Part print with two shaded views. Sizes in mm from the minimum x, y, z corner. Give positions to 0.01 mm unless a question says otherwise; leave off trailing zeros. Loops run counter-clockwise (first coordinate to the right, second up) from the corner with the lowest first, then second, coordinate; pieces in that order, holes last. Notation, with made-up numbers: (78.5, 27.25) -> (103.5, 27.25) arc R28 cw to (103.5, 64.25) -> close; hole circle Ø1 at (85.5, 68). An arc over 180 degrees is marked (long way). One line per question, with ' | ' between items. Start each with the question number.
(1) Slice it at D-D, the plane x = 38. Write the cut outline in (y, z), then the cut area to 3 significant figures.
(2) Drill centre lines: L1, parallel to Z at x = 22.5, y = 1.2; L2, parallel to Z at x = 7, y = 1.4; L3, parallel to Z at x = 42, y = 2.1 (1 decimal). Where is each one in solid material? Low to high. Write a range as from..to.
(3) Slice it at B-B, the plane y = 2.45. Write the cut outline in (x, z).
(4) Slice it at C-C, the plane z = 7. Write the cut outline in (x, y) (1 decimal).
(5) Flat gauge pins, fed straight in: pin 1 Ø6.5 at (x, z) = (22.5, 8.55) entering from +Y; pin 2 Ø1 at (x, y) = (10, 2.5) entering from +Z. Where does each tip first touch, or does it go through?
(6) Slice it at A-A, the plane x = 22.5. Write the cut outline in (y, z).
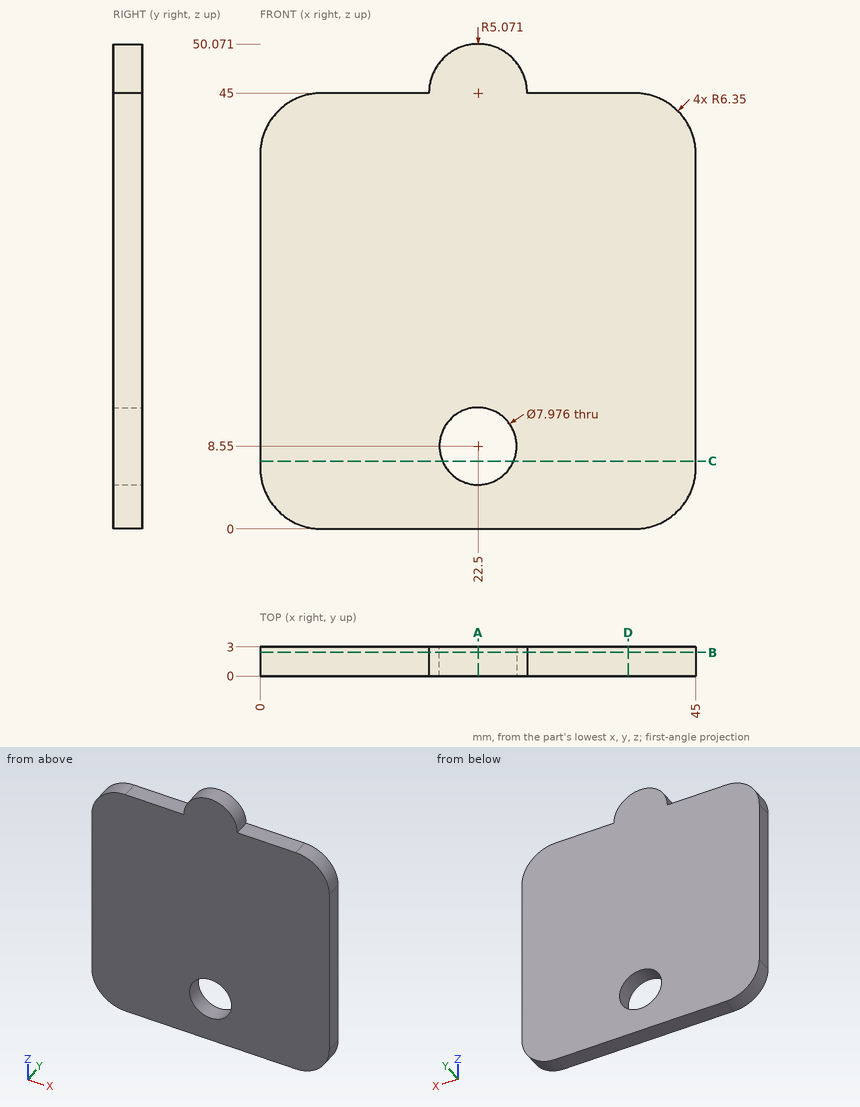
Final values:
1) outline: (0, 0) -> (3, 0) -> (3, 45) -> (0, 45) -> close | area: 135 mm2
2) L1: 0..4.56, 12.54..50.07 | L2: 0..45 | L3: 1..44
3) outline: (0, 6.35) arc R6.35 ccw to (6.35, 0) -> (38.65, 0) arc R6.35 ccw to (45, 6.35) -> (45, 38.65) arc R6.35 ccw to (38.65, 45) -> (27.57, 45) arc R5.07 ccw to (17.43, 45) -> (6.35, 45) arc R6.35 ccw to (0, 38.65) -> close; hole circle Ø7.98 at (22.5, 8.55)
4) outline: (0, 0) -> (18.8, 0) -> (18.8, 3) -> (0, 3) -> close; (26.2, 0) -> (45, 0) -> (45, 3) -> (26.2, 3) -> close
5) pin 1: through | pin 2: z = 45
6) outline: (0, 0) -> (3, 0) -> (3, 4.56) -> (0, 4.56) -> close; (0, 12.54) -> (3, 12.54) -> (3, 50.07) -> (0, 50.07) -> close
